Check sheet for the modelled part. Datum: model origin and axes. Units: mm. Round coordinates to 2 decimals unless told otherwise and drop trailing zeros. Loops run counter-clockwise (first coordinate to the right, second up) from the corner with the lowest first, then second, coordinate; pieces in that order, holes last. Notation, with made-up numbers: (69, -38.75) - (79, -38.75) arc R19 cw to (79, -28.75) - close; hole circle Ø2 at (17.5, -21). An arc over 180 degrees is marked (long way). Return JSON: item names as keys, results as strings.
from build123d import *

# Parameters (mm, degrees)
SKETCH1_R          = 6.4
EXTRUDE1_DEPTH     = 3
SKETCH2_R          = 8
EXTRUDE2_DEPTH     = 5
SKETCH3_R          = 4
CUT_EXTRUDE1_DEPTH = 33.062439084


with BuildPart() as part:
    # Sketch1 → Extrude1 (new body)
    with BuildSketch(Plane.XY):
        with Locations((0, -22)):
            Circle(SKETCH1_R)
    extrude(amount=-EXTRUDE1_DEPTH)

    # Sketch2 → Extrude2 (add)
    with BuildSketch(Plane(origin=(0, 0, -3), x_dir=(-1, 0, 0), z_dir=(0, 0, -1))):
        with Locations((0, -22)):
            Circle(SKETCH2_R)
    extrude(amount=EXTRUDE2_DEPTH)

    # Sketch3 → Cut-Extrude1 (cut, through all)
    with BuildSketch(Plane.XY):
        with Locations((0, -22)):
            Circle(SKETCH3_R)
    extrude(amount=-CUT_EXTRUDE1_DEPTH, mode=Mode.SUBTRACT)


solid = part.part
Q1. Sectioned sample at D-D (y = -17.25). Enter the section's corners in (x, z), plus the area to 3 significant figures.
Answer key:
{"outline": "(-6.44, -8) - (6.44, -8) - (6.44, -3) - (4.29, -3) - (4.29, 0) - (-4.29, 0) - (-4.29, -3) - (-6.44, -3) - close", "area": "90.1 mm²"}
Q2. Depth check by flat-ended pin: P1, Ø2, axis at y = -23.5, z = -4.5, coming from the -X side; P2, Ø1, axis at y = -21, z = -2, coming from the -X side; P3, Ø1, axis at x = 2, z = -1, coming from the -Y side. Enter the tip coordinate at first touch or a pass-through.
Answer key:
{"P1": "stops at x = -7.98", "P2": "stops at x = -6.38", "P3": "stops at y = -28.22"}
Q3. Scan lines: probe 1 along Y at (x, z) = (0, -1.75); probe 2 along Z at (x, y) = (-5.25, -17.25); probe 3 along Y at (x, z) = (2.5, -1.5). Record each from-to range of solid material in increasing order. Write a range as [from, to].
Answer key:
{"probe 1": "y = [-28.4, -26], [-18, -15.6]", "probe 2": "z = [-8, -3]", "probe 3": "y = [-27.89, -25.12], [-18.88, -16.11]"}
Q4. Draft check along X on faces 1 (the face through (0, -15, -3)), 2 (the face through (-0.521, -18.034, -3.944)), 3 (the face through (-1.387, -28.248, -1.479)). Enter one of: released by +X, released by -X, zero draft, split by the parting line, or undercut.
Answer key:
{"face 1": "zero draft", "face 2": "undercut", "face 3": "split by the parting line"}
Q5. Sectioned sample at A-A (y = -22). Enter the section's corners in (x, z).
Answer key:
{"outline": "(-8, -8) - (-4, -8) - (-4, 0) - (-6.4, 0) - (-6.4, -3) - (-8, -3) - close; (4, -8) - (8, -8) - (8, -3) - (6.4, -3) - (6.4, 0) - (4, 0) - close"}
Q6. Sectioned sample at B-B (x = -2). Enter the section's corners in (y, z), plus the area to 3 significant figures.
Answer key:
{"outline": "(-29.75, -8) - (-25.46, -8) - (-25.46, 0) - (-28.08, 0) - (-28.08, -3) - (-29.75, -3) - close; (-18.54, -8) - (-14.25, -8) - (-14.25, -3) - (-15.92, -3) - (-15.92, 0) - (-18.54, 0) - close", "area": "58.5 mm²"}
Q7. Sectioned sample at C-C (z = -2). Enter the section's corners in (x, y), plus the area to 3 significant figures.
Answer key:
{"outline": "circle Ø12.8 at (0, -22); hole circle Ø8 at (0, -22)", "area": "78.4 mm²"}
